from build123d import *

# Parameters (mm, degrees)
SKETCH2_W           = 160
SKETCH2_H           = 160
BOSS_EXTRUDE2_DEPTH = 6
SKETCH3_W           = 26.5
SKETCH3_H           = 48.5
BOSS_EXTRUDE3_DEPTH = 32
SKETCH4_W           = 20.5
SKETCH4_H           = 42.5
CUT_EXTRUDE2_DEPTH  = 29
SKETCH5_R           = 4
BOSS_EXTRUDE4_DEPTH = 8
CUT_EXTRUDE3_DEPTH  = 8
SKETCH7_R           = 1.25
CUT_EXTRUDE4_DEPTH  = 10


with BuildPart() as part:
    # Sketch2 → Boss-Extrude2 (new body)
    with BuildSketch(Plane(origin=(0, 0, 0), x_dir=(1, 0, 0), z_dir=(0, 1, 0))):
        Rectangle(SKETCH2_W, SKETCH2_H)
    extrude(amount=BOSS_EXTRUDE2_DEPTH)

    # Sketch3 → Boss-Extrude3 (add)
    with BuildSketch(Plane(origin=(0, 0, 0), x_dir=(1, 0, 0), z_dir=(0, 1, 0))):
        with Locations((-66.75, 55.75)):
            Rectangle(SKETCH3_W, SKETCH3_H)
        with Locations((66.75, 55.75)):
            Rectangle(SKETCH3_W, SKETCH3_H)
        with Locations((66.75, -55.75)):
            Rectangle(SKETCH3_W, SKETCH3_H)
        with Locations((-66.75, -55.75)):
            Rectangle(SKETCH3_W, SKETCH3_H)
    extrude(amount=BOSS_EXTRUDE3_DEPTH)

    # Sketch4 → Cut-Extrude2 (cut)
    with BuildSketch(Plane(origin=(0, 0, 0), x_dir=(1, 0, 0), z_dir=(0, 1, 0))):
        with Locations((-66.75, 55.75)):
            Rectangle(SKETCH4_W, SKETCH4_H)
        with Locations((66.75, 55.75)):
            Rectangle(SKETCH4_W, SKETCH4_H)
        with Locations((66.75, -55.75)):
            Rectangle(SKETCH4_W, SKETCH4_H)
        with Locations((-66.75, -55.75)):
            Rectangle(SKETCH4_W, SKETCH4_H)
    extrude(amount=CUT_EXTRUDE2_DEPTH, mode=Mode.SUBTRACT)

    # Sketch5 → Boss-Extrude4 (add)
    with BuildSketch(Plane(origin=(0, 32, 0), x_dir=(1, 0, 0), z_dir=(0, 1, 0))):
        with Locations(Location((-66.75, 66.5, 0), (0, 0, 270))):
            Circle(SKETCH5_R)
        with Locations(Location((66.75, 66.5, 0), (0, 0, 90))):
            Circle(SKETCH5_R)
        with Locations(Location((66.75, -66.5, 0), (0, 0, 270))):
            Circle(SKETCH5_R)
        with Locations(Location((-66.75, -66.5, 0), (0, 0, 90))):
            Circle(SKETCH5_R)
    extrude(amount=BOSS_EXTRUDE4_DEPTH)

    # Sketch6 → Cut-Extrude3 (cut)
    with BuildSketch(Plane.XY.offset(80)):
        Polygon((-73, 27), (-61, 27), (-61, 22), (-62.5, 22), (-62.5, 2), (-71.5, 2), (-71.5, 22), (-73, 22), align=None)
        Polygon((73, 22), (73, 27), (61, 27), (61, 22), (62.5, 22), (62.5, 2), (71.5, 2), (71.5, 22), align=None)
    cut_extrude3 = extrude(amount=-CUT_EXTRUDE3_DEPTH, mode=Mode.SUBTRACT)

    # Mirror1: Cut-Extrude3 across plane
    add(cut_extrude3.mirror(Plane.XY), mode=Mode.SUBTRACT)

    # Sketch7 → Cut-Extrude4 (cut)
    with BuildSketch(Plane(origin=(0, 6, 0), x_dir=(1, 0, 0), z_dir=(0, 1, 0))):
        with Locations(Location((-60.85, 0, 0), (0, 0, 270))):
            Circle(SKETCH7_R)
        with Locations(Location((0, 60.85, 0), (0, 0, 270))):
            Circle(SKETCH7_R)
        with Locations(Location((60.85, 0, 0), (0, 0, 270))):
            Circle(SKETCH7_R)
        with Locations(Location((0, -60.85, 0), (0, 0, 270))):
            Circle(SKETCH7_R)
    extrude(amount=-CUT_EXTRUDE4_DEPTH, mode=Mode.SUBTRACT)


solid = part.part
Geometry: final body of the model. Coordinates: model frame, mm. A direction names the side the tool comes from. Coordinates: 2 decimals unless noted, no trailing zeros. Order: outer loops, then holes, each group sorted by start corner. A loop starts at its lowest first (then second) coordinate and runs counter-clockwise, first axis right, second up. Notation, with made-up numbers: (32.5, -10.75) - (68.5, -10.75) arc R9 cw to (68.5, 1.25) - close; hole circle Ø10 at (75.5, 53). An arc over 180 degrees is marked (long way). Use one line per item in the form item = value.
1) Section A-A (x = 66.75). State how many separate pieces and enclosed holes the cut face has, then the cut area to 3 significant figures.
Solutions:
separate_pieces = 3
enclosed_holes = 0
area = 995 mm^2
2) Set-up query: faces 5 (the face through (77, 14, 56)), 6 (the face through (63.201, 35.944, 68.346)), 7 (the face through (-53.5, 19, 56)), 8 (the face through (-67, 19, -31.5)). Return all of +Z, -Z, +X, -X, +Y, -Y with unobstructed straight access to the full face (end or side cutting, diameter ignored); none if empty.
Solutions:
face_5 = -Y
face_6 = +Y
face_7 = +Z, -Z, +Y
face_8 = +X, -X, +Y
3) Mould query, pull axis X, two halves, no side actions, for faces 1 (the face through (53.5, 19, -55)), 2 (the face through (-67, 29, 55)), 3 (the face through (-67, 40, 67)), 4 (the face through (-80, 5, 1)). Classes: +X half, -X half, draft (parallel to the pull), parting line (faces both ways), or undercut.
Solutions:
face_1 = undercut
face_2 = undercut
face_3 = draft
face_4 = -X half
4) Section B-B (z = 66.5). Return loops of the section in (x, y).
Solutions:
outline = (-80, 0) - (-77, 0) - (-77, 29) - (-56.5, 29) - (-56.5, 0) - (56.5, 0) - (56.5, 29) - (77, 29) - (77, 0) - (80, 0) - (80, 32) - (70.75, 32) - (70.75, 40) - (62.75, 40) - (62.75, 32) - (53.5, 32) - (53.5, 6) - (-53.5, 6) - (-53.5, 32) - (-62.75, 32) - (-62.75, 40) - (-70.75, 40) - (-70.75, 32) - (-80, 32) - close
5) Section D-D (x = 15.5). Return loops of the section in (y, z).
Solutions:
outline = (0, -80) - (6, -80) - (6, 80) - (0, 80) - close
6) Ray query, L1, parallel to X at y = 2.6, z = 0; L2, parallel to X at y = 25.5, z = 65.5; L3, parallel to X at y = 3.6, z = -60.85. Return the intervals inside material, ascending.
Solutions:
L1 = -80 to -62.1, -59.6 to 59.6, 62.1 to 80
L2 = -80 to -77, -56.5 to -53.5, 53.5 to 56.5, 77 to 80
L3 = -80 to -77, -56.5 to -1.25, 1.25 to 56.5, 77 to 80
7) Pin query (flat end, axial travel): pin 1 (8 mm diameter, centred on x = -26, z = -41.5, fed in from +Y); pin 2 (16.5 mm diameter, centred on x = 68, z = 65, fed in from -Y); pin 3 (1.2 mm diameter, centred on x = 72.5, z = -79, fed in from +Y). Return the tip coordinate at first contact, or that it passes through.
Solutions:
pin_1 = 6
pin_2 = 29
pin_3 = 32
